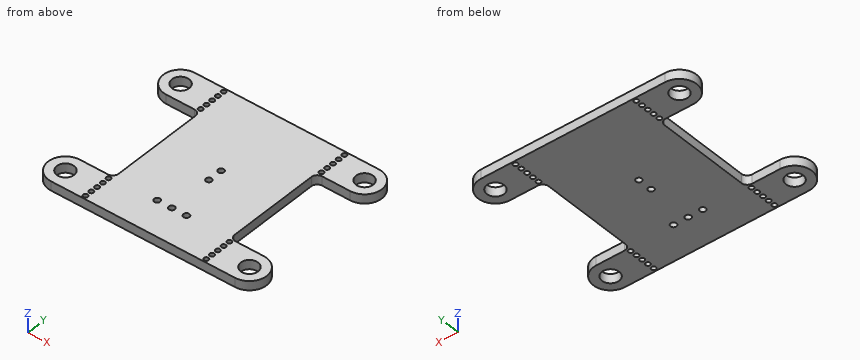
Autodesk Inventor part; units mm, degrees
ref_plane "BoardFrontPlane" through (0, 0, 0) normal (0, 0, 1) x (1, 0, 0)
ref_plane "YZ Plane" through (0, 0, 0) normal (1, 0, 0) x (0, 1, 0)
ref_plane "XZ Plane" through (0, 0, 0) normal (0, 1, 0) x (-1, 0, 0)
ref_plane "BoardFrontPlane" through (0, 0, 0) normal (0, 0, 1) x (1, 0, 0)
sketch "Sketch1" plane through (0, 0, 0) normal (0, 0, 1) x (1, 0, 0)
  line L0 (19.5, 24.465) -> (47.5, 24.465)
  line L1 (47.5, 24.465) -> (51.5, 24.465)
  arc A0 (51.5, 24.465) -> (51.5, 30.465) centre (51.5, 27.465) ccw
  line L2 (51.5, 30.465) -> (46.6, 30.4645)
  arc A1 (45.5997, 31.4679) -> (46.6, 30.4645) centre (46.6001, 31.4649) ccw
  line L3 (45.5997, 31.4679) -> (45.6001, 47.4621)
  arc A2 (46.6004, 48.4653) -> (45.6001, 47.4621) centre (46.6004, 47.465) ccw
  line L4 (46.6004, 48.4653) -> (51.5004, 48.465)
  arc A3 (51.5004, 48.465) -> (51.5004, 54.465) centre (51.5004, 51.465) ccw
  line L5 (51.5004, 54.465) -> (47.5004, 54.465)
  line L6 (47.5004, 54.465) -> (19.5004, 54.465)
  arc A4 (19.5004, 54.465) -> (19.5004, 48.465) centre (19.5004, 51.465) ccw
  line L7 (19.5004, 48.465) -> (24.4004, 48.4655)
  arc A5 (25.4007, 47.4621) -> (24.4004, 48.4655) centre (24.4003, 47.4651) ccw
  line L8 (25.4007, 47.4621) -> (25.4003, 31.4679)
  arc A6 (24.4, 30.4647) -> (25.4003, 31.4679) centre (24.4, 31.465) ccw
  line L9 (24.4, 30.4647) -> (19.5, 30.465)
  arc A7 (19.5, 30.465) -> (19.5, 24.465) centre (19.5, 27.465) ccw
extrude "BoardOutline" add sketch "Sketch1" along normal blind 1.5954
sketch "img_Top" plane through (0, 0, 1.5954) normal (0, 0, 1) x (1, 0, 0)
  line L0 (16.5, 54.465) -> (54.5017, 54.465) construction
  line L1 (54.5017, 54.465) -> (54.5017, 24.465) construction
  line L2 (54.5017, 24.465) -> (16.5, 24.465) construction
  line L3 (16.5, 24.465) -> (16.5, 54.465) construction
decal "Decal_Top"
sketch "img_Bottom" plane through (0, 0, -1.5954) normal (0, 0, -1) x (1, 0, 0)
  line L0 (16.5, -24.465) -> (54.5017, -24.465) construction
  line L1 (54.5017, -24.465) -> (54.5017, -54.465) construction
  line L2 (54.5017, -54.465) -> (16.5, -54.465) construction
  line L3 (16.5, -54.465) -> (16.5, -24.465) construction
decal "Decal_Bottom"
sketch "Sketch4" plane through (0, 0, 1.5954) normal (0, 0, 1) x (1, 0, 0)
  point P0 (35.5, 40.735)
hole "Q1-2" at (35.5, 40.735, 1.5954) direction (0, 0, -1) diameter 1.016 end through all
sketch "Sketch5" plane through (0, 0, 1.5954) normal (0, 0, 1) x (1, 0, 0)
  point P0 (35.5, 38.195)
hole "Q1-1" at (35.5, 38.195, 1.5954) direction (0, 0, -1) diameter 1.016 end through all
sketch "Sketch6" plane through (0, 0, 1.5954) normal (0, 0, 1) x (1, 0, 0)
  point P0 (46.0004, 53.865)
hole "Free-6_WBTLOXPK" at (46.0004, 53.865, 1.5954) direction (0, 0, -1) diameter 0.8 end through all
sketch "Sketch7" plane through (0, 0, 1.5954) normal (0, 0, 1) x (1, 0, 0)
  point P0 (46.0004, 52.665)
hole "Free-5_XIOJIJXP" at (46.0004, 52.665, 1.5954) direction (0, 0, -1) diameter 0.8 end through all
sketch "Sketch8" plane through (0, 0, 1.5954) normal (0, 0, 1) x (1, 0, 0)
  point P0 (46.0004, 51.465)
hole "Free-4_DJTYKPAA" at (46.0004, 51.465, 1.5954) direction (0, 0, -1) diameter 0.8 end through all
sketch "Sketch9" plane through (0, 0, 1.5954) normal (0, 0, 1) x (1, 0, 0)
  point P0 (46.0004, 50.265)
hole "Free-3_AXXACNQN" at (46.0004, 50.265, 1.5954) direction (0, 0, -1) diameter 0.8 end through all
sketch "Sketch10" plane through (0, 0, 1.5954) normal (0, 0, 1) x (1, 0, 0)
  point P0 (46.0004, 49.065)
hole "Free-2_AOCKDCBY" at (46.0004, 49.065, 1.5954) direction (0, 0, -1) diameter 0.8 end through all
sketch "Sketch11" plane through (0, 0, 1.5954) normal (0, 0, 1) x (1, 0, 0)
  point P0 (51.5004, 51.465)
hole "Free-1_DASBMRFB" at (51.5004, 51.465, 1.5954) direction (0, 0, -1) diameter 3 end through all
sketch "Sketch12" plane through (0, 0, 1.5954) normal (0, 0, 1) x (1, 0, 0)
  point P0 (25.0004, 53.865)
hole "Free-6_NIMWPQYT" at (25.0004, 53.865, 1.5954) direction (0, 0, -1) diameter 0.8 end through all
sketch "Sketch13" plane through (0, 0, 1.5954) normal (0, 0, 1) x (1, 0, 0)
  point P0 (25.0004, 52.665)
hole "Free-5_XNHNLNST" at (25.0004, 52.665, 1.5954) direction (0, 0, -1) diameter 0.8 end through all
sketch "Sketch14" plane through (0, 0, 1.5954) normal (0, 0, 1) x (1, 0, 0)
  point P0 (25.0004, 51.465)
hole "Free-4_FETUHRKC" at (25.0004, 51.465, 1.5954) direction (0, 0, -1) diameter 0.8 end through all
sketch "Sketch15" plane through (0, 0, 1.5954) normal (0, 0, 1) x (1, 0, 0)
  point P0 (25.0004, 50.265)
hole "Free-3_DMTDOSJH" at (25.0004, 50.265, 1.5954) direction (0, 0, -1) diameter 0.8 end through all
sketch "Sketch16" plane through (0, 0, 1.5954) normal (0, 0, 1) x (1, 0, 0)
  point P0 (25.0004, 49.065)
hole "Free-2_TMPFYMJS" at (25.0004, 49.065, 1.5954) direction (0, 0, -1) diameter 0.8 end through all
sketch "Sketch17" plane through (0, 0, 1.5954) normal (0, 0, 1) x (1, 0, 0)
  point P0 (19.5004, 51.465)
hole "Free-1_WWOKCKJL" at (19.5004, 51.465, 1.5954) direction (0, 0, -1) diameter 3 end through all
sketch "Sketch18" plane through (0, 0, 1.5954) normal (0, 0, 1) x (1, 0, 0)
  point P0 (51.5, 27.465)
hole "Free-1_SGRFTGBA" at (51.5, 27.465, 1.5954) direction (0, 0, -1) diameter 3 end through all
sketch "Sketch19" plane through (0, 0, 1.5954) normal (0, 0, 1) x (1, 0, 0)
  point P0 (46, 29.865)
hole "Free-2_AUMGPVUD" at (46, 29.865, 1.5954) direction (0, 0, -1) diameter 0.8 end through all
sketch "Sketch20" plane through (0, 0, 1.5954) normal (0, 0, 1) x (1, 0, 0)
  point P0 (46, 28.665)
hole "Free-3_HPVJLOHR" at (46, 28.665, 1.5954) direction (0, 0, -1) diameter 0.8 end through all
sketch "Sketch21" plane through (0, 0, 1.5954) normal (0, 0, 1) x (1, 0, 0)
  point P0 (46, 27.465)
hole "Free-4_DQHIBCUL" at (46, 27.465, 1.5954) direction (0, 0, -1) diameter 0.8 end through all
sketch "Sketch22" plane through (0, 0, 1.5954) normal (0, 0, 1) x (1, 0, 0)
  point P0 (46, 26.265)
hole "Free-5_OUJHCFEU" at (46, 26.265, 1.5954) direction (0, 0, -1) diameter 0.8 end through all
sketch "Sketch23" plane through (0, 0, 1.5954) normal (0, 0, 1) x (1, 0, 0)
  point P0 (46, 25.065)
hole "Free-6_RFLYKSPV" at (46, 25.065, 1.5954) direction (0, 0, -1) diameter 0.8 end through all
sketch "Sketch24" plane through (0, 0, 1.5954) normal (0, 0, 1) x (1, 0, 0)
  point P0 (25, 25.065)
hole "Free-6_SWLXYYKK" at (25, 25.065, 1.5954) direction (0, 0, -1) diameter 0.8 end through all
sketch "Sketch25" plane through (0, 0, 1.5954) normal (0, 0, 1) x (1, 0, 0)
  point P0 (25, 26.265)
hole "Free-5_RJKXWDHV" at (25, 26.265, 1.5954) direction (0, 0, -1) diameter 0.8 end through all
sketch "Sketch26" plane through (0, 0, 1.5954) normal (0, 0, 1) x (1, 0, 0)
  point P0 (25, 27.465)
hole "Free-4_KOIALDYT" at (25, 27.465, 1.5954) direction (0, 0, -1) diameter 0.8 end through all
sketch "Sketch27" plane through (0, 0, 1.5954) normal (0, 0, 1) x (1, 0, 0)
  point P0 (25, 28.665)
hole "Free-3_NUADKFXF" at (25, 28.665, 1.5954) direction (0, 0, -1) diameter 0.8 end through all
sketch "Sketch28" plane through (0, 0, 1.5954) normal (0, 0, 1) x (1, 0, 0)
  point P0 (25, 29.865)
hole "Free-2_KKFAPUKC" at (25, 29.865, 1.5954) direction (0, 0, -1) diameter 0.8 end through all
sketch "Sketch29" plane through (0, 0, 1.5954) normal (0, 0, 1) x (1, 0, 0)
  point P0 (19.5, 27.465)
hole "Free-1_BKUUHACL" at (19.5, 27.465, 1.5954) direction (0, 0, -1) diameter 3 end through all
sketch "Sketch30" plane through (0, 0, 1.5954) normal (0, 0, 1) x (1, 0, 0)
  point P0 (32.96, 30.465)
hole "P1-1" at (32.96, 30.465, 1.5954) direction (0, 0, -1) diameter 1.04 end through all
sketch "Sketch31" plane through (0, 0, 1.5954) normal (0, 0, 1) x (1, 0, 0)
  point P0 (35.5, 30.465)
hole "P1-2" at (35.5, 30.465, 1.5954) direction (0, 0, -1) diameter 1.04 end through all
sketch "Sketch32" plane through (0, 0, 1.5954) normal (0, 0, 1) x (1, 0, 0)
  point P0 (38.04, 30.465)
hole "P1-3" at (38.04, 30.465, 1.5954) direction (0, 0, -1) diameter 1.04 end through all
properties part number "Dual PMT Controller - Light Interlock_BOARD"
The listing builds one solid part. Answer for the finished solid, in the listing's coordinates (mm). Give positions to 0.01 mm unless a question says otherwise; leave off trailing zeros. Write each loop counter-clockwise with the first axis right and the second up, starting at its lowest first coordinate (ties: lowest second). Pieces come first, ordered by that corner, then holes.
Item 1: Find the intervals of material crossed by line 1 along Y through (x, z) = (23.5, 0.8) (3 decimals); line 2 along Y through (x, z) = (35.5, 0.5) (3 decimals); line 3 along Y through (x, z) = (32.96, 0.3) (3 decimals), in increasing order.
Item 2: Section C-C, the plane y = 43 is taken. Write down the section's boundary in (x, z), plus the area to 3 significant figures.
Item 3: Section A-A, the plane x = 32.96 is taken. Write down the section's boundary in (y, z) (3 decimals).
Item 4: Flat-ended cylindrical pins translate along their axes: P1, Ø1.7, axis at x = 32.96, y = 30.465, coming from the +Z side; P2, Ø1.8, axis at x = 19.5, y = 27.465, coming from the -Z side; P3, Ø0.5, axis at y = 38, z = 1, coming from the -X side. Find the tip coordinate at first contact, or state that the pin passes through.
Item 5: Section B-B, the plane x = 49.5 is taken. Write down the section's boundary in (y, z) (3 decimals), plus the area to 3 significant figures.
Completed:
1. line 1: y = 24.465 to 30.465, 48.465 to 54.465
1. line 2: y = 24.465 to 29.945, 30.985 to 37.687, 38.703 to 40.227, 41.243 to 54.465
1. line 3: y = 24.465 to 29.945, 30.985 to 54.465
2. outline: (25.4, 0) - (45.6, 0) - (45.6, 1.6) - (25.4, 1.6) - close
2. area: 32.2 mm2
3. outline: (24.465, 0) - (29.945, 0) - (29.945, 1.595) - (24.465, 1.595) - close; (30.985, 0) - (54.465, 0) - (54.465, 1.595) - (30.985, 1.595) - close
4. P1: stops at z = 1.6
4. P2: passes through
4. P3: stops at x = 25.4
5. outline: (24.465, 0) - (30.465, 0) - (30.465, 1.595) - (24.465, 1.595) - close; (48.465, 0) - (54.465, 0) - (54.465, 1.595) - (48.465, 1.595) - close
5. area: 19.1 mm2
